```python
from build123d import *

# Parameters (mm, degrees)
F0_W     = 63
F0_H     = 40
F1_DEPTH = 75
F2_DEPTH = 25


with BuildPart() as f1:
    # F0 (on Front) → F1 (new body)
    with BuildSketch(Plane.XZ):
        with Locations((-48.5, 5)):
            Rectangle(F0_W, F0_H)
        Polygon((80, 25), (17, 25), (17, -15), (27.937743758, -15), (27.937743758, 0), (80, 0), align=None)
        with BuildLine():
            Line((17, 25), (0, 25))
            Line((0, 25), (0, -5))
            ThreePointArc((0, -5), (7.0710678119, -7.9289321881), (10, -15))
            Line((10, -15), (17, -15))
            Line((17, -15), (17, 25))
        make_face()
        with BuildLine():
            Line((0, 25), (-17, 25))
            Line((-17, 25), (-17, -15))
            Line((-17, -15), (-10, -15))
            ThreePointArc((-10, -15), (-7.0710678119, -7.9289321881), (0, -5))
            Line((0, -5), (0, 25))
        make_face()
        with Locations((-48.5, -35)):
            Rectangle(F0_W, F0_H)
        Polygon((27.937743758, -15), (17, -15), (17, -55), (80, -55), (80, -30), (27.937743758, -30), align=None)
        with BuildLine():
            Line((-10, -15), (-17, -15))
            Line((-17, -15), (-17, -55))
            Line((-17, -55), (0, -55))
            Line((0, -55), (0, -25))
            ThreePointArc((0, -25), (-7.0710678119, -22.0710678119), (-10, -15))
        make_face()
        with BuildLine():
            Line((17, -55), (17, -15))
            Line((17, -15), (10, -15))
            ThreePointArc((10, -15), (7.0710678119, -22.0710678119), (0, -25))
            Line((0, -25), (0, -55))
            Line((0, -55), (17, -55))
        make_face()
    extrude(amount=F1_DEPTH)

    # F2 (add): a face of the model
    f2_faces = [f1.faces().sort_by_distance(p)[0] for p in [
        (0, -37.5, 25),
    ]]
    extrude(f2_faces, amount=F2_DEPTH)


solid = f1.part
```
Input: part model. Units: mm. Frame: model coordinates. A direction names the side the tool comes from. Coordinates: 2 decimals unless noted, no trailing zeros. Loops run counter-clockwise (first coordinate to the right, second up) from the corner with the lowest first, then second, coordinate; pieces in that order, holes last. Notation, with made-up numbers: (66.5, 15) - (91.5, 15) arc R28 ccw to (91.5, 33) - close; hole circle Ø2 at (0, 29.25). An arc over 180 degrees is marked (long way). Answer in a Markdown table with one row per item.
(1) Mould query, pull axis Z, two halves, no side actions, for faces 1 (the face through (-1, -37, -55)), 2 (the face through (54, -37, -30)), 3 (the face through (54, -37, 0)), 4 (the face through (1, 0, -3)). Classes: pulls with the +Z half, pulls with the -Z half, needs draft (parallel to the pull), parting line crosses it, or undercut.
Model answer:
| item | result |
|---|---|
| face 1 | pulls with the -Z half |
| face 2 | undercut |
| face 3 | undercut |
| face 4 | needs draft |
(2) Set-up query: faces 5 (the face through (1, -75, -3)), 6 (the face through (27.938, -37, -15)). Return all of +Z, -Z, +X, -X, +Y, -Y with unobstructed straight access to the full face (end or side cutting, diameter ignored); none if empty.
Model answer:
| item | result |
|---|---|
| face 5 | +Z, -Z, +X, -X, -Y |
| face 6 | +X, +Y, -Y |
(3) Pin query (flat end, axial travel): P1, Ø5, axis at y = -25.5, z = -10.5, coming from the +X side. Return the tip coordinate at first contact, or that it passes through.
Model answer:
| item | result |
|---|---|
| P1 | stops at x = 27.94 |
(4) Cut plane B-B on x = 30.5. Output: boundary loops of the cut face in (y, z), plus the area to 4 significant figures.
Model answer:
| item | result |
|---|---|
| outline | (-75, -55) - (0, -55) - (0, -30) - (-75, -30) - close; (-75, 0) - (0, 0) - (0, 50) - (-75, 50) - close |
| area | 5,625 mm² |
(5) Cut plane C-C on x = -7. Output: boundary loops of the cut face in (y, z), plus the area to 3 significant figures.
Model answer:
| item | result |
|---|---|
| outline | (-75, -55) - (0, -55) - (0, -22.14) - (-75, -22.14) - close; (-75, -7.86) - (0, -7.86) - (0, 50) - (-75, 50) - close |
| area | 6,800 mm² |
(6) Cut plane A-A on y = -23.5. Output: boundary loops of the cut face in (x, z).
Model answer:
| item | result |
|---|---|
| outline | (-80, -55) - (80, -55) - (80, -30) - (27.94, -30) - (27.94, 0) - (80, 0) - (80, 50) - (-80, 50) - close; hole circle Ø20 at (0, -15) |
(7) Material intervals for L1, parallel to Z at x = 30, y = -32; L2, parallel to X at y = -36, z = -27; L3, parallel to X at y = -35.5, z = -22, sorted ascending. Write a range as from..to.
Model answer:
| item | result |
|---|---|
| L1 | z = -55..-30, 0..50 |
| L2 | x = -80..27.94 |
| L3 | x = -80..-7.14, 7.14..27.94 |
